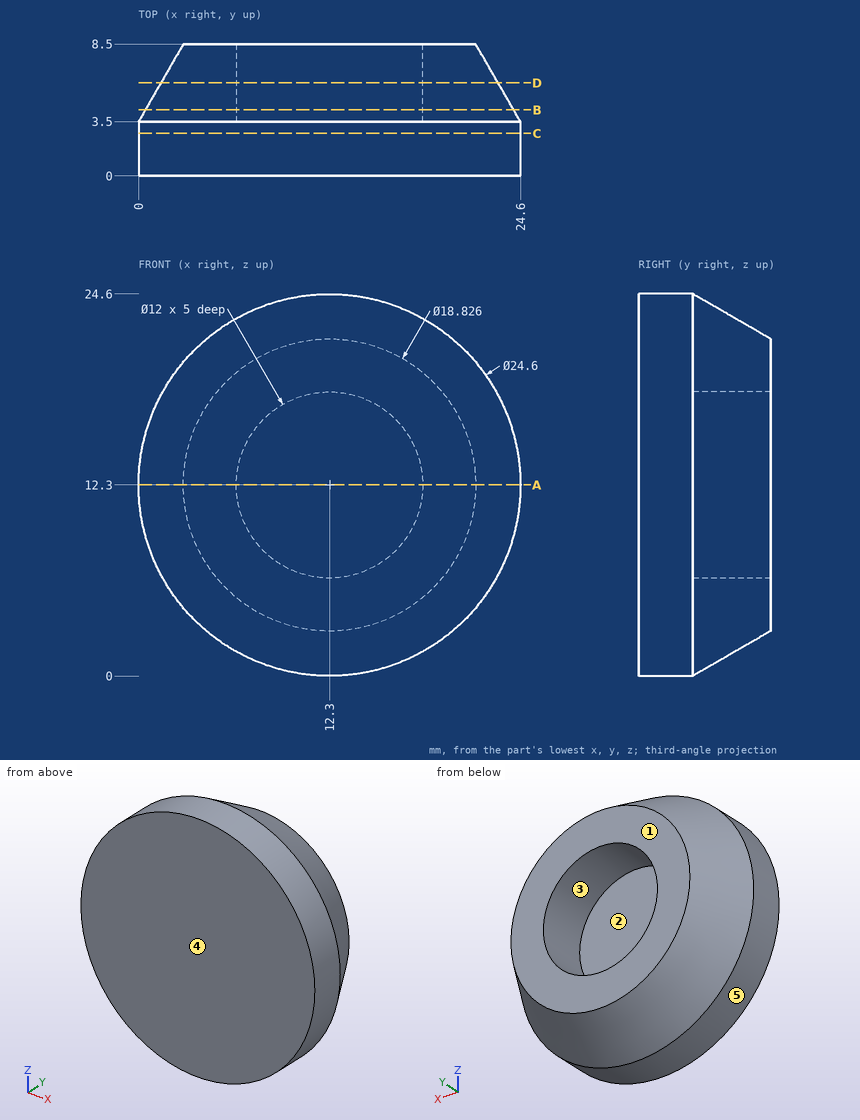
Geometry: see drawing. Coordinates: mm, zero at the bounding-box minimum. A direction names the side the tool comes from. Coordinates: 2 decimals unless noted, no trailing zeros. Loops run counter-clockwise (first coordinate to the right, second up) from the corner with the lowest first, then second, coordinate; pieces in that order, holes last.
(1) Material intervals for probe 1 along X at (y, z) = (6.15, 12.3); probe 2 along Y at (x, z) = (12.75, 17); probe 3 along Z at (x, y) = (12.3, 5.9) (1 decimal), sorted ascending.
(2) Section A-A on z = 12.3. Return the cut outline in (x, y), then the cut area to 3 significant figures.
(3) Section D-D on y = 6. Return the cut outline in (x, z).
(4) Section C-C on y = 2.75. Return the cut outline in (x, z), then the cut area to 3 significant figures.
(5) First-contact query: pin 1 Ø2 at (x, y) = (17.5, 1.5) entering from +Z; pin 2 Ø1.5 at (x, y) = (9, 3.5) entering from -Z; pin 3 Ø4 at (x, y) = (18, 7.5) entering from +Z (1 decimal). Flat tips, straight axial feed; report the tip coordinate or a pass-through.
(6) Set-up query: the marked faces 1 and 2. Return all of +Z, -Z, +X, -X, +Y, -Y with unobstructed straight access to the full face (end or side cutting, diameter ignored); none if empty.
(7) Section B-B on y = 4.25. Return the cut outline in (x, z), then the cut area to 3 significant figures.
(8) Pull-direction query (X, two-part tool) for the marked faces 3, 4 and 5; classes: released by +X, released by -X, zero draft, split by the parting line, or undercut.
Data:
1. probe 1: x = 1.53 to 6.3, 18.3 to 23.07
1. probe 2: y = 0 to 3.5
1. probe 3: z = 1.4 to 6.3, 18.3 to 23.2
2. outline: (0, 0) - (24.6, 0) - (24.6, 3.5) - (21.71, 8.5) - (18.3, 8.5) - (18.3, 3.5) - (6.3, 3.5) - (6.3, 8.5) - (2.89, 8.5) - (0, 3.5) - close
2. area: 135 mm2
3. outline: circle Ø21.71 at (12.3, 12.3); hole circle Ø12 at (12.3, 12.3)
4. outline: circle Ø24.6 at (12.3, 12.3)
4. area: 475 mm2
5. pin 1: stops at z = 23.86
5. pin 2: stops at z = 0.27
5. pin 3: stops at z = 22.2
6. face 1: +Z, -Z, +X, -X, +Y
6. face 2: +Y
7. outline: circle Ø23.73 at (12.3, 12.3); hole circle Ø12 at (12.3, 12.3)
7. area: 329 mm2
8. face 3: undercut
8. face 4: zero draft
8. face 5: split by the parting line
